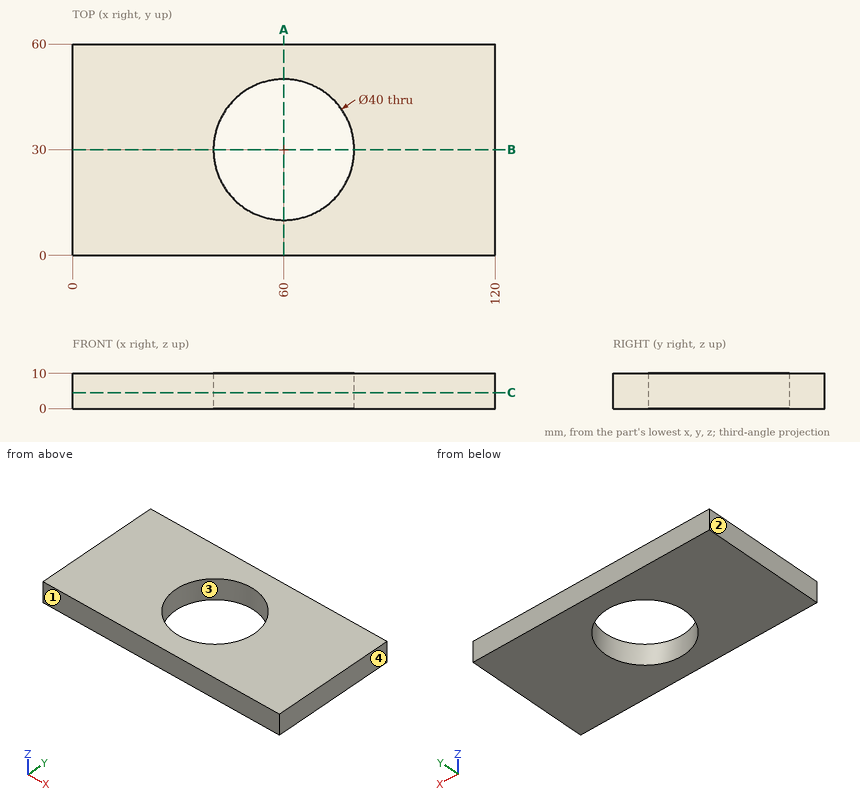
Input: dimensioned drawing with shaded views. Units: mm. Origin: part minimum x, y, z. Round coordinates to 2 decimals unless told otherwise and drop trailing zeros. Loops run counter-clockwise (first coordinate to the right, second up) from the corner with the lowest first, then second, coordinate; pieces in that order, holes last. Notation, with made-up numbers: (-23, -29) -> (5, -29) arc R15 cw to (5, -13) -> close; hole circle Ø5 at (-3.75, -12.75). An arc over 180 degrees is marked (long way). Answer as a JSON object with one key per item and string values. Group by question number.
1) Section query B-B on y = 30. Output: boundary loops of the cut face in (x, z).
2) Section query C-C on z = 4.5. Output: boundary loops of the cut face in (x, y), plus the area to 3 significant figures.
3) Draft query along X for the marked faces 1, 2, 3 and 4. Return one class per face: +X half, -X half, draft (parallel to the pull), parting line (faces both ways), or undercut.
4) Ray query, L1, parallel to Y at x = 60, z = 4.5; L2, parallel to X at y = 37, z = 2.25 (3 decimals); L3, parallel to X at y = 16, z = 7.5. Return the intervals inside material, ascending.
5) Section query A-A on x = 60. Output: boundary loops of the cut face in (y, z), plus the area to 3 significant figures.
Reply:
{
 "1": {"outline": "(0, 0) -> (40, 0) -> (40, 10) -> (0, 10) -> close; (80, 0) -> (120, 0) -> (120, 10) -> (80, 10) -> close"},
 "2": {"outline": "(0, 0) -> (120, 0) -> (120, 60) -> (0, 60) -> close; hole circle Ø40 at (60, 30)", "area": "5,940 mm2"},
 "3": {"face 1": "draft", "face 2": "-X half", "face 3": "undercut", "face 4": "+X half"},
 "4": {"L1": "y = 0 to 10, 50 to 60", "L2": "x = 0 to 41.265, 78.735 to 120", "L3": "x = 0 to 45.72, 74.28 to 120"},
 "5": {"outline": "(0, 0) -> (10, 0) -> (10, 10) -> (0, 10) -> close; (50, 0) -> (60, 0) -> (60, 10) -> (50, 10) -> close", "area": "200 mm2"}
}
